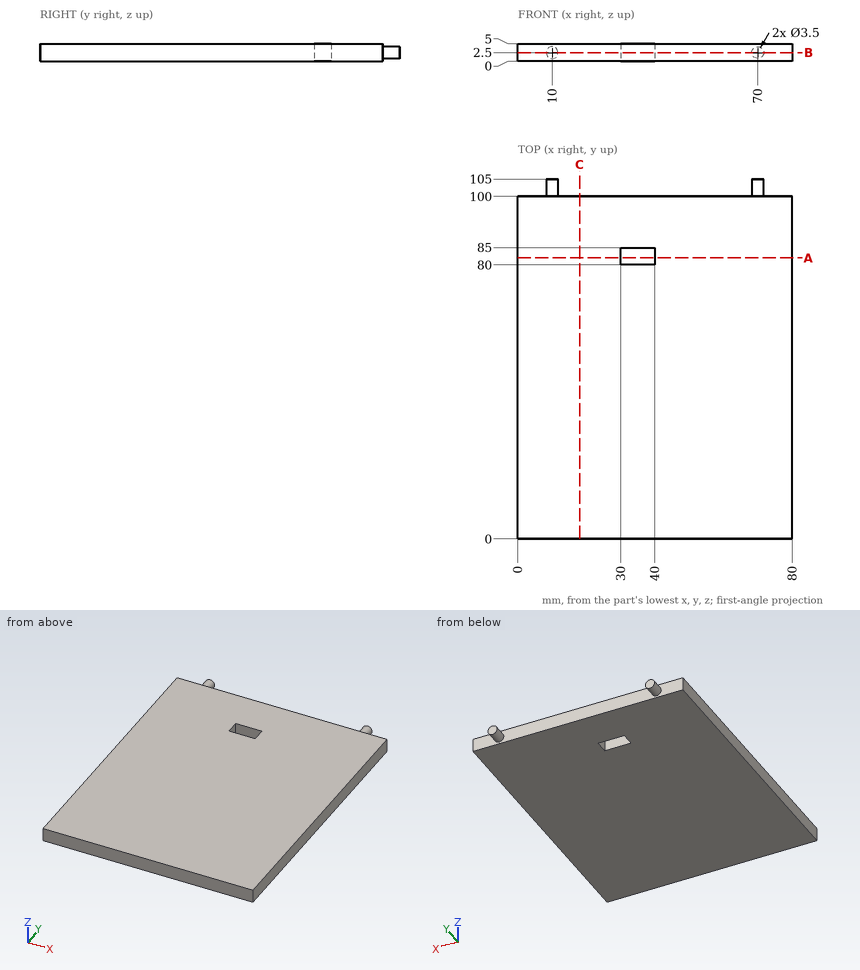
Study the drawing (mm; zero at the part's minimum x, y, z) and answer. Coordinates: 2 decimals unless noted, no trailing zeros. Write each loop counter-clockwise with the first axis right and the second up, starting at its lowest first coordinate (ties: lowest second). Pieces come first, ordered by that corner, then holes. Notation, with made-up numbers: (81.5, -38) - (114.5, -38) arc R32 ccw to (114.5, -8) - close; hole circle Ø4 at (-17, 80.5). An arc over 180 degrees is marked (long way). Answer as a JSON object with one key per item and string values. Group by question number.
1. This flat-tipped pin is pushed along its axis until it touches: P1, Ø3, axis at x = 64.5, z = 4.5, coming from the +Y side. Where does it stop, or does it pass through?
2. A cutting plane is placed at B-B (z = 2.5). Determine the outline of the cut face in (x, y), plus the area to 4 significant figures.
3. Consider L1, parallel to Y at x = 38, z = 2.35; L2, parallel to Y at x = 27, z = 3.55; L3, parallel to X at y = 82.5, z = 4.35. Determine where each line is inside the solid, lowest interval first. Write a range as [from, to].
4. A cutting plane is placed at A-A (y = 82). Determine the outline of the cut face in (x, z).
5. A cutting plane is placed at C-C (x = 18). Determine the outline of the cut face in (y, z).
Worked out:
{
 "1": {"P1": "stops at y = 100"},
 "2": {"outline": "(0, 0) - (80, 0) - (80, 100) - (71.75, 100) - (71.75, 105) - (68.25, 105) - (68.25, 100) - (11.75, 100) - (11.75, 105) - (8.25, 105) - (8.25, 100) - (0, 100) - close; hole (30, 80) - (40, 80) - (40, 85) - (30, 85) - close", "area": "7,985 mm²"},
 "3": {"L1": "y = [0, 80], [85, 100]", "L2": "y = [0, 100]", "L3": "x = [0, 30], [40, 80]"},
 "4": {"outline": "(0, 0) - (30, 0) - (30, 5) - (0, 5) - close; (40, 0) - (80, 0) - (80, 5) - (40, 5) - close"},
 "5": {"outline": "(0, 0) - (100, 0) - (100, 5) - (0, 5) - close"}
}
